```python
from build123d import *

# Parameters (mm, degrees)
F0_W        = 25
F0_H        = 24
F1_DEPTH    = 15
F2_T        = -1.2
F3_DEPTH    = 25
F4_W        = 22.6
F4_H        = 7.1360613033
F5_DEPTH    = 25
F6_T4_DEPTH = 22.6
F7_R        = 5
F8_SIZE     = 8
F9_R        = 5
F10_R       = 1
F11_SIZE    = 7


# Not quite as in the source:
# - a fillet or chamfer that OpenCascade refuses, or shapes differently, is made with other operations: its cross-section is extruded or revolved along the edge and cut away or added


with BuildPart() as f1:
    # F0 (on Top) → F1 (new body)
    with BuildSketch(Plane.XY):
        with Locations((-29.1051699208, 12)):
            Rectangle(F0_W, F0_H)
    extrude(amount=F1_DEPTH)

    # F2
    f2_openings = [f1.faces().sort_by_distance(p)[0] for p in [
        (-29.10517, 12, 15),
    ]]
    offset(amount=F2_T, openings=f2_openings)

    # F3 (cut): a face of the model
    f3_faces = [f1.faces().sort_by_distance(p)[0] for p in [
        (-29.1051699208, 1.2, 8.1),
    ]]
    extrude(f3_faces, amount=-F3_DEPTH, mode=Mode.SUBTRACT)

    # F4 (on face) → F5 (cut)
    with BuildSketch(Plane.XZ.offset(-22.8)):
        with Locations((-29.1051699208, 11.4319693483)):
            Rectangle(F4_W, F4_H)
    extrude(amount=-F5_DEPTH, mode=Mode.SUBTRACT)

    # F6: chamfer of 10 on 1 edges, made by hand


with BuildPart() as f6_tool2:
    # F6_s3 → F6_t4 (new body)
    with BuildSketch(Plane.YZ.offset(-17.8051699208)):
        Polygon((22.8, 11.2), (12.8, 1.2), (22.8, 1.2), align=None)
    extrude(amount=-F6_T4_DEPTH)

    split(bisect_by=Plane.XY.offset(7.8639386967), keep=Keep.BOTTOM)


with BuildPart() as f1_1:
    add(f1.part)

    # F6_t1: union F6_tool2
    add(f6_tool2.part)

    # F7
    f7_edges = [f1_1.edges().sort_by_distance(p)[0] for p in [
        (-29.10517, 12.8, 1.2),
        (-17.20517, 24, 15),
        (-41.00517, 24, 15),
    ]]
    fillet(f7_edges, radius=F7_R)

    # F8
    f8_edges = [f1_1.edges().sort_by_distance(p)[0] for p in [
        (-41.00517, 0, 15),
        (-17.20517, 0, 15),
    ]]
    chamfer(f8_edges, length=F8_SIZE)

    # F9
    f9_edges = [f1_1.edges().sort_by_distance(p)[0] for p in [
        (-41.00517, 8, 15),
        (-41.00517, 0, 7),
        (-17.20517, 0, 7),
        (-17.20517, 8, 15),
    ]]
    fillet(f9_edges, radius=F9_R)

    # F10
    f10_edges = [f1_1.edges().sort_by_distance(p)[0] for p in [
        (-40.40517, 5.364466, 1.2),
        (-17.80517, 5.364466, 1.2),
        (-17.80517, 12.642349, 1.580602),
        (-17.80517, 16.864202, 5.264202),
        (-40.40517, 16.864202, 5.264202),
        (-40.40517, 12.642349, 1.580602),
    ]]
    fillet(f10_edges, radius=F10_R)

    # F11
    f11_edges = [f1_1.edges().sort_by_distance(p)[0] for p in [
        (-29.10517, 24, 0),
    ]]
    chamfer(f11_edges, length=F11_SIZE)


solid = f1_1.part
```
Read the model definition and answer for the solid it produces. Units are mm, in the model's axes. A direction names the side the tool comes from. Give positions to 0.01 mm unless a question says otherwise; leave off trailing zeros. Write each loop counter-clockwise with the first axis right and the second up, starting at its lowest first coordinate (ties: lowest second). Pieces come first, ordered by that corner, then holes. Notation, with made-up numbers: M 12.25,45 L 48.25,45 A32 ccw 48.25,72 Z; hole C 50,31 d6. An arc over 180 degrees is marked long. Put each result on its own line as item: value. Start each with the question number.
1. Consider line 1 along X through (y, z) = (8, 8.75); line 2 along Z through (x, y) = (-39.5, 8); line 3 along Z through (x, y) = (-29, 23). Determine where each line is inside the solid, lowest interval first.
2. For a pull along X with two mould halves and no side action, classify faces 1 (the cylindrical face through (-17.2, 0.39, 6.87)), 2 (the flat face through (-29, 5, 1.2)), 3 (the flat face through (-16.605, 12, 7)) as released by +X, released by -X, zero draft, split by the parting line, or undercut.
3. The part is cut by section B-B, the plane z = 11.5. Give the vertices of the cut face in (x, y).
4. The part is cut by section D-D, the plane y = 9.5. Give the vertices of the cut face in (x, z).
5. The part is cut by section A-A, the plane x = -25.75. Give the vertices of the cut face in (y, z).
6. The part is cut by section C-C, the plane y = 7. Give the vertices of the cut face in (x, z), and give its area (3 significant figures).
7. Each of these flat-tipped pins is pushed along its axis until it touches: pin 1 Ø1.5 at (x, z) = (-31.5, 5.5) entering from -Y; pin 2 Ø8 at (x, y) = (-36, 17) entering from +Z; pin 3 Ø1 at (x, y) = (-38.5, 14) entering from +Z. Where does it stop, or does it pass through?
8. Which of the six approach directions +Z, -Z, +X, -X, +Y, -Y give full straight-line access (tool end or side, diameter ignored) to faces 4 (the cylindrical face through (-41, 23, 13)), 5 (the cylindrical face through (-40.104, 5.289, 1.485)), 6 (the flat face through (-29, 22, 7.864))?
Final values:
1. line 1: x = -41.61 to -40.41, -17.81 to -16.61
1. line 2: z = 0 to 1.2
1. line 3: z = 6 to 7.86
2. face 1: zero draft
2. face 2: undercut
2. face 3: released by +X
3. outline: M -41.61,4.5 L -40.41,4.5 L -40.41,23.77 L -41.61,23.77 Z; M -17.81,4.5 L -16.61,4.5 L -16.61,23.77 L -17.81,23.77 Z
4. outline: M -41.61,0 L -16.61,0 L -16.61,14.97 L -17.81,14.97 L -17.81,2.2 A1 cw -18.81,1.2 L -39.41,1.2 A1 cw -40.41,2.2 L -40.41,14.97 L -41.61,14.97 Z
5. outline: M 0,0 L 17,0 L 24,7 L 24,7.86 L 19.46,7.86 L 14.26,2.66 A5 cw 10.73,1.2 L 0,1.2 Z
6. outline: M -41.61,0 L -16.61,0 L -16.61,13.95 L -17.81,13.95 L -17.81,2.2 A1 cw -18.81,1.2 L -39.41,1.2 A1 cw -40.41,2.2 L -40.41,13.95 L -41.61,13.95 Z
6. area: 61.0 mm²
7. pin 1: stops at y = 16.35
7. pin 2: stops at z = 7.86
7. pin 3: stops at z = 2.9
8. face 4: +Z, +X, -X, +Y
8. face 5: +Z, -Y
8. face 6: +Z, +Y, -Y
